Can you work these out from the model? Positions are in its coordinate system, mm. A direction names the side the tool comes from. Round coordinates to 2 decimals unless told otherwise and drop trailing zeros. Loops run counter-clockwise (first coordinate to the right, second up) from the corner with the lowest first, then second, coordinate; pieces in that order, holes last.
(1) Will these pins go through, and if not, where does the flat tip stop? pin 1 Ø2.5 at (x, y) = (40.5, 11.5) entering from -Z; pin 2 Ø5 at (x, y) = (-19.5, -5) entering from -Z.
(2) Thinking about a two-plate mould opening in Y: for faces 1 (the face through (45.42, 17.36, 1.48)), 2 (the face through (-37, 9, 2)), 3 (the face through (20, 34, 1)), 4 (the face through (-20.932, 4.406, 1.479)), which applies, released by +Y, released by -Y, zero draft, split by the parting line, or undercut?
(3) I want a section at B-B on z = 1.3. Give the number of separate pieces and of enclosed holes in the cut face, plus the area to 3 significant figures.
(4) I want a section at C-C on y = 18. Write out the boundary of the cut face in (x, z).
(5) I want a section at A-A on x = 12. Write out the boundary of the cut face in (y, z), plus the area to 3 significant figures.
(6) Which directions (+Z, -Z, +X, -X, +Y, -Y) give clear straight access to the entire face, cutting with the end or side of a thin tool? Please do faces 5 (the face through (67, 0, 2)), 6 (the face through (7, 10, 0)).
(7) I want a section at D-D on x = 46.25. Write out the boundary of the cut face in (y, z).
(8) If I drill on line 1 along Y through (x, z) = (12, 1.5); line 2 along Y through (x, z) = (34.5, 1.3); line 3 along Y through (x, z) = (52.5, 1.15), over which ranges is the centre line in solid material (lowest first)?
from build123d import *

# Parameters (mm, degrees)
SKETCH_1_W          = 74
SKETCH_1_H          = 30
EXTRUDE_1_DEPTH     = 3
SKETCH_2_R          = 1.55
SKETCH_2_R_2        = 2.1
CUT_EXTRUDE_1_DEPTH = 3
SKETCH_3_W          = 30
SKETCH_3_H          = 30
SKETCH_3_R          = 11.25
SKETCH_3_R_2        = 1.3
EXTRUDE_2_DEPTH     = 3
SKETCH_4_W          = 74
SKETCH_4_H          = 19
EXTRUDE_3_DEPTH     = 3
SKETCH_5_R          = 1.05
CUT_EXTRUDE_2_DEPTH = 10
SKETCH_6_R          = 1.05
CUT_EXTRUDE_4_DEPTH = 10
SKETCH_7_W          = 30
SKETCH_7_H          = 3
EXTRUDE_4_DEPTH     = 19
SKETCH_10_W         = 8
SKETCH_10_H         = 19
EXTRUDE_6_DEPTH     = 3
SKETCH_11_R         = 1.05
CUT_EXTRUDE_5_DEPTH = 10
SKETCH_12_W         = 72.681959433
SKETCH_12_H         = 19
EXTRUDE_7_DEPTH     = 3
SKETCH_13_R         = 1.05
CUT_EXTRUDE_7_DEPTH = 3


with BuildPart() as part:
    # 草图1 → 凸台-拉伸1 (new body)
    with BuildSketch(Plane.XY):
        Rectangle(SKETCH_1_W, SKETCH_1_H)
    extrude(amount=EXTRUDE_1_DEPTH)

    # 草图2 → 切除-拉伸1 (cut)
    with BuildSketch(Plane(origin=(0, 0, 0), x_dir=(-1, 0, 0), z_dir=(0, 0, -1))):
        with Locations((-34.5, 5)):
            Circle(SKETCH_2_R)
        with Locations((-34.5, -5)):
            Circle(SKETCH_2_R)
        with Locations((-19.5, 5)):
            Circle(SKETCH_2_R)
        with Locations((-19.5, -5)):
            Circle(SKETCH_2_R)
        with Locations((-12, 10)):
            Circle(SKETCH_2_R_2)
        with Locations((12, 10)):
            Circle(SKETCH_2_R_2)
        with Locations((-12, -10)):
            Circle(SKETCH_2_R_2)
        with Locations((12, -10)):
            Circle(SKETCH_2_R_2)
        with Locations((34.5, 5)):
            Circle(SKETCH_2_R)
        with Locations((34.5, -5)):
            Circle(SKETCH_2_R)
        with Locations((19.5, 5)):
            Circle(SKETCH_2_R)
        with Locations((19.5, -5)):
            Circle(SKETCH_2_R)
    extrude(amount=-CUT_EXTRUDE_1_DEPTH, mode=Mode.SUBTRACT)

    # 草图3 → 凸台-拉伸2 (add)
    with BuildSketch(Plane.XY.offset(3)):
        with Locations((52, 0)):
            Rectangle(SKETCH_3_W, SKETCH_3_H)
        with Locations((52, 0)):
            Circle(SKETCH_3_R, mode=Mode.SUBTRACT)
        with Locations((40.5, 11.5)):
            Circle(SKETCH_3_R_2, mode=Mode.SUBTRACT)
        with Locations((63.5, 11.5)):
            Circle(SKETCH_3_R_2, mode=Mode.SUBTRACT)
        with Locations((40.5, -11.5)):
            Circle(SKETCH_3_R_2, mode=Mode.SUBTRACT)
        with Locations((63.5, -11.5)):
            Circle(SKETCH_3_R_2, mode=Mode.SUBTRACT)
    extrude(amount=-EXTRUDE_2_DEPTH)

    # 草图4 → 凸台-拉伸3 (add, through all)
    with BuildSketch(Plane.XY.offset(3)):
        with Locations((0, 24.5)):
            Rectangle(SKETCH_4_W, SKETCH_4_H)
    extrude(amount=-EXTRUDE_3_DEPTH)

    # 草图5 → 切除-拉伸2 (cut)
    with BuildSketch(Plane.XY.offset(3)):
        with Locations((-21.5, 31.5)):
            Circle(SKETCH_5_R)
        with Locations((-21.5, 16.5)):
            Circle(SKETCH_5_R)
        with Locations((-11.5, 31.5)):
            Circle(SKETCH_5_R)
        with Locations((-11.5, 16.5)):
            Circle(SKETCH_5_R)
        with Locations((27, 31.5)):
            Circle(SKETCH_5_R)
        with Locations((17, 31.5)):
            Circle(SKETCH_5_R)
        with Locations((17, 16.5)):
            Circle(SKETCH_5_R)
        with Locations((27, 16.5)):
            Circle(SKETCH_5_R)
    extrude(amount=-CUT_EXTRUDE_2_DEPTH, mode=Mode.SUBTRACT)

    # 草图6 → 切除-拉伸4 (cut)
    with BuildSketch(Plane.XY.offset(3)):
        with Locations((-20.5, 30)):
            Circle(SKETCH_6_R)
        with Locations((-12.5, 30)):
            Circle(SKETCH_6_R)
        with Locations((-12.5, 18)):
            Circle(SKETCH_6_R)
        with Locations((-20.5, 18)):
            Circle(SKETCH_6_R)
        with Locations((18, 30)):
            Circle(SKETCH_6_R)
        with Locations((26, 30)):
            Circle(SKETCH_6_R)
        with Locations((26, 18)):
            Circle(SKETCH_6_R)
        with Locations((18, 18)):
            Circle(SKETCH_6_R)
    extrude(amount=-CUT_EXTRUDE_4_DEPTH, mode=Mode.SUBTRACT)

    # 草图7 → 凸台-拉伸4 (add, through all)
    with BuildSketch(Plane(origin=(0, 15, 0), x_dir=(1, 0, 0), z_dir=(0, 1, 0))):
        with Locations((52, -1.5)):
            Rectangle(SKETCH_7_W, SKETCH_7_H)
    extrude(amount=EXTRUDE_4_DEPTH)

    # 草图10 → 凸台-拉伸6 (add)
    with BuildSketch(Plane(origin=(0, 0, 0), x_dir=(-1, 0, 0), z_dir=(0, 0, -1))):
        with Locations((-71, 24.5)):
            Rectangle(SKETCH_10_W, SKETCH_10_H)
    extrude(amount=-EXTRUDE_6_DEPTH)

    # 草图11 → 切除-拉伸5 (cut)
    with BuildSketch(Plane.XY.offset(3)):
        with Locations((59.75, 30)):
            Circle(SKETCH_11_R)
        with Locations((67.75, 30)):
            Circle(SKETCH_11_R)
        with Locations((59.75, 18)):
            Circle(SKETCH_11_R)
        with Locations((67.75, 18)):
            Circle(SKETCH_11_R)
    extrude(amount=-CUT_EXTRUDE_5_DEPTH, mode=Mode.SUBTRACT)

    # 草图12 → 凸台-拉伸7 (add)
    with BuildSketch(Plane.XY):
        with Locations((-0.659020283, 24.5)):
            Rectangle(SKETCH_12_W, SKETCH_12_H)
    extrude(amount=EXTRUDE_7_DEPTH)

    # 草图13 → 切除-拉伸7 (cut)
    with BuildSketch(Plane.XY):
        with Locations((46.25, 30)):
            Circle(SKETCH_13_R)
        with Locations((46.25, 18)):
            Circle(SKETCH_13_R)
        with Locations((38.25, 18)):
            Circle(SKETCH_13_R)
        with Locations((38.25, 30)):
            Circle(SKETCH_13_R)
    extrude(amount=CUT_EXTRUDE_7_DEPTH, mode=Mode.SUBTRACT)


solid = part.part
Filled sheet:
1. pin 1: passes through
1. pin 2: stops at z = 0
2. face 1: undercut
2. face 2: zero draft
2. face 3: released by +Y
2. face 4: undercut
3. separate pieces: 1
3. enclosed holes: 25
3. area: 4,690 mm2
4. outline: (-37, 0) - (37.2, 0) - (37.2, 3) - (-37, 3) - close; (39.3, 0) - (45.2, 0) - (45.2, 3) - (39.3, 3) - close; (47.3, 0) - (58.7, 0) - (58.7, 3) - (47.3, 3) - close; (60.8, 0) - (66.7, 0) - (66.7, 3) - (60.8, 3) - close; (68.8, 0) - (75, 0) - (75, 3) - (68.8, 3) - close
5. outline: (-15, 0) - (-12.1, 0) - (-12.1, 3) - (-15, 3) - close; (-7.9, 0) - (7.9, 0) - (7.9, 3) - (-7.9, 3) - close; (12.1, 0) - (34, 0) - (34, 3) - (12.1, 3) - close
5. area: 122 mm2
6. face 5: +Z, -Z, +X, -Y
6. face 6: -Z, +X, -X, +Y, -Y
7. outline: (-15, 0) - (-9.67, 0) - (-9.67, 3) - (-15, 3) - close; (9.67, 0) - (16.95, 0) - (16.95, 3) - (9.67, 3) - close; (19.05, 0) - (28.95, 0) - (28.95, 3) - (19.05, 3) - close; (31.05, 0) - (34, 0) - (34, 3) - (31.05, 3) - close
8. line 1: y = -15 to -12.1, -7.9 to 7.9, 12.1 to 34
8. line 2: y = -15 to -6.55, -3.45 to 3.45, 6.55 to 34
8. line 3: y = -15 to -11.24, 11.24 to 34
